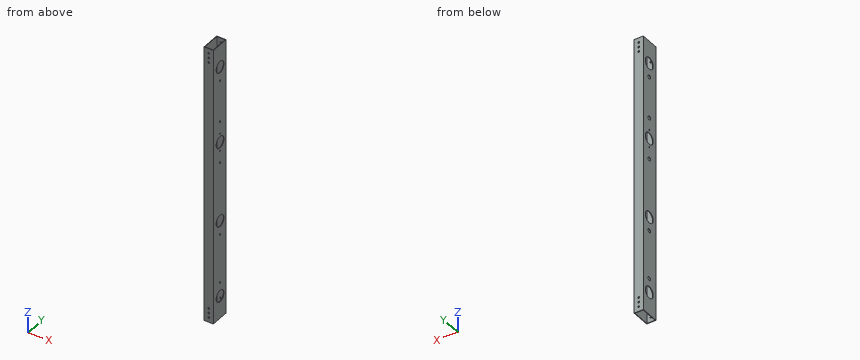
Autodesk Inventor part; units mm, degrees
ref_plane "YZ Plane" through (0, 0, 0) normal (1, 0, 0) x (0, 1, 0)
ref_plane "XZ Plane" through (0, 0, 0) normal (0, 1, 0) x (-1, 0, 0)
ref_plane "XY Plane" through (0, 0, 0) normal (0, 0, 1) x (1, 0, 0)
sketch "Sketch1" plane through (0, 0, 0) normal (1, 0, 0) x (0, 1, 0)
  line L0 (25.4, -381) -> (-25.4, -381)
  line L1 (-25.4, -381) -> (-25.4, 381)
  line L2 (-25.4, 381) -> (25.4, 381)
  line L3 (25.4, 381) -> (25.4, -381)
  line L4 (25.4, -381) -> (-25.4, 381) construction
  line L5 (-25.4, -381) -> (25.4, 381) construction
  circle A0 centre (1.5875, -319.0875) radius 15.875
  line L6 (0, -381) -> (0, -205.8364) construction
  circle A1 centre (1.5875, -280.9875) radius 2.4892
  circle A2 centre (1.5875, -280.9875) radius 5.2705
  circle A3 centre (-1.5875, 0) radius 15.875
  line L7 (0, 0) -> (48.0139, 0) construction
  circle A4 centre (1.5875, 319.0875) radius 15.875
  circle A5 centre (1.5875, 280.9875) radius 2.4892
  circle A6 centre (1.5875, 280.9875) radius 5.2705
  circle A7 centre (1.5875, -319.0875) radius 76.2 construction
  circle A8 centre (-1.5875, 0) radius 76.2 construction
  circle A9 centre (1.5875, 319.0875) radius 76.2 construction
  circle A10 centre (-1.5875, -23.8125) radius 2.0193
  circle A11 centre (19.0347, -11.9063) radius 2.0193
  circle A12 centre (19.0347, 11.9062) radius 2.0193
  circle A13 centre (-1.5875, 23.8125) radius 2.0193
  circle A14 centre (-22.2097, 11.9062) radius 2.0193 construction
  circle A15 centre (-22.2097, -11.9063) radius 2.0193 construction
  circle A16 centre (-1.5875, -57.15) radius 2.4892
  circle A17 centre (-1.5875, -57.15) radius 5.2705
  circle A18 centre (-1.5875, 57.15) radius 2.4892
  circle A19 centre (-1.5875, 57.15) radius 5.2705
  circle A20 centre (1.5875, -109.5375) radius 15.875
  circle A21 centre (1.5875, -147.6375) radius 2.4892
  circle A22 centre (1.5875, -147.6375) radius 5.2705
  line L8 (1.5875, 280.9875) -> (1.5875, 319.0875) construction
  line L9 (1.5875, -109.5375) -> (1.5875, -147.6375) construction
  circle A23 centre (1.5875, 85.725) radius 2.0193
  circle A24 centre (1.5875, 52.3875) radius 2.4892
  circle A25 centre (1.5875, 52.3875) radius 5.2705
  circle A26 centre (1.5875, 166.6875) radius 2.4892
  circle A27 centre (1.5875, 166.6875) radius 5.2705
  circle A28 centre (1.5875, 133.35) radius 2.0193
  line L10 (1.5875, 133.35) -> (1.5875, 85.725) construction
  line L11 (-1.5875, 23.8125) -> (-1.5875, -23.8125) construction
  line L12 (1.5875, 166.6875) -> (1.5875, 52.3875) construction
  line L13 (-1.5875, 57.15) -> (-1.5875, -57.15) construction
  circle A29 centre (1.5875, 109.5375) radius 15.875
  line L14 (25.4, 381) -> (-25.4, 381) construction
  line L15 (-25.4, 381) -> (-25.4, 406.4) construction
  line L16 (-25.4, 406.4) -> (25.4, 406.4) construction
  line L17 (25.4, 406.4) -> (25.4, 381) construction
  line L18 (25.4, 404.8125) -> (-25.4, 404.8125) construction
  line L19 (25.4, 401.6375) -> (-25.4, 401.6375) construction
  point P0 (0, 0)
  point P1 (1.5875, 1.5875)
  point P2 (1.5875, -19.5792)
  point P3 (3.2385, -19.5792)
  point P4 (1.5875, -19.5792)
  dimension "d0" = 762
  dimension "d1" = 50.8
  dimension "d2" = 31.75
  dimension "d4" = 10.541
  dimension "d5" = 4.9784
  dimension "d6" = 1.5875
  dimension "d7" = 1.5875
  dimension "d8" = 38.1
  dimension "d9" = 319.0875
  dimension "d10" = 152.4
  dimension "d13" = 4.0386
  dimension "d16" = 360
  dimension "d18" = 4.9784
  dimension "d19" = 10.541
  dimension "d20" = 114.3
  dimension "d21" = 47.625
  dimension "d22" = 3.1903
  dimension "d26" = 4.0386
  dimension "d28" = 4.9784
  dimension "d29" = 10.541
  dimension "d33" = 360
  dimension "d35" = 219.075
  dimension "d36" = 209.55
  dimension "d58" = 25.4
  dimension "d59" = 1.5875
  dimension "d60" = 3.175
extrude "Extrusion1" add sketch "Sketch1" along normal mid plane 25.4 contours L0 L1 L2 L3 | A2 | A3 | A6 | A10 | A11 | A12 | A13 | A16 | A17 | A18 A25 | A18 A25 A19 A24 | A25 A18 | A18 A25 A19 | A25 A19 A24 | A22 | A27
sketch "Sketch2" plane through (-12.7, -25.4, -381) normal (0, 0, -1) x (-1, 0, 0)
  line L0 (0, 50.8) -> (-25.4, 50.8)
  line L1 (-25.4, 0) -> (-25.4, 50.8)
  line L2 (0, 50.8) -> (0, 0)
  line L3 (-23.8125, 49.2125) -> (-1.5875, 49.2125)
  line L4 (-1.5875, 49.2125) -> (-1.5875, 1.5875)
  line L5 (-1.5875, 1.5875) -> (-23.8125, 1.5875)
  line L6 (-23.8125, 1.5875) -> (-23.8125, 49.2125)
  line L7 (0, 0) -> (-25.4, 0)
  point P0 (-12.7, 25.4)
  dimension "d23" = 1.5875
extrude "Extrusion2" cut sketch "Sketch2" against normal through all contours L3 L4 L5 L6
sketch "Sketch3" plane through (-12.7, 25.4, 381) normal (0, 1, 0) x (1, 0, 0)
  line L0 (0, 762) -> (25.4, 762)
  line L1 (0, 762) -> (25.4, 762)
  line L2 (12.7, 762) -> (12.7, 749.3)
  circle A0 centre (12.7, 749.3) radius 2.4892
  circle A1 centre (12.7, 736.6) radius 2.4892
  circle A2 centre (12.7, 723.9) radius 2.4892
  line L3 (12.7, 381) -> (42.3415, 381) construction
  circle A3 centre (12.7, 12.7) radius 2.4892
  circle A4 centre (12.7, 25.4) radius 2.4892
  circle A5 centre (12.7, 38.1) radius 2.4892
  dimension "d37" = 12.7
  dimension "d38" = 4.9784
  dimension "d41" = 12.7
extrude "Extrusion3" cut sketch "Sketch3" against normal through all
sketch "Sketch4" plane through (-12.7, 0, 0) normal (-1, 0, 0) x (0, 0, 1)
  circle A0 centre (280.9875, 1.5875) radius 2.4892
  circle A1 centre (-280.9875, 1.5875) radius 2.4892
  circle A2 centre (52.3875, 1.5875) radius 2.4892
  circle A3 centre (166.6875, 1.5875) radius 2.4892
  circle A4 centre (-147.6375, 1.5875) radius 2.4892
  point P0 (0, 0)
  point P1 (57.15, -1.5875)
hole "Hole1" at (-12.7, 1.5875, 280.9875) at (-12.7, 1.5875, 52.3875) at (-12.7, 1.5875, 166.6875) at (-12.7, 1.5875, -280.9875) at (-12.7, 1.5875, -147.6375) direction (1, 0, 0) diameter 4.9784 depth 25.4 tip angle 118 counterbore diameter 10.541 counterbore depth 4.826
equation "\"d7\" = d6"
properties part number "VersaChassis Drive Rail Template" material "Aluminum"
CAD build for the part. Positions are in the model's coordinates, mm. Round coordinates to 2 decimals unless told otherwise and drop trailing zeros. Order: outer loops, then holes, each group sorted by start corner. A loop starts at its lowest first (then second) coordinate and runs counter-clockwise, first axis right, second up. Notation, with made-up numbers: (12, 6.5) - (46, 6.5) arc R15 ccw to (46, 16.5) - close; hole circle Ø7 at (-10.5, -19.5). An arc over 180 degrees is marked (long way). Answer in a Markdown table with one row per item. Add a question column.
(1) Drop flat-ended pins along their axis: pin 1 Ø4 at (y, z) = (0.5, -145.5) entering from +X; pin 2 Ø5.5 at (y, z) = (1.59, 166.69) entering from -X. Give the stop position or say it passes through.
(2) Probe L1, parallel to Y at x = -11, z = 141; L2, parallel to X at y = -7.5, z = 64.5; L3, parallel to X at y = -24.15, z = 355.6. List the from-to ranges inside material, lowest first. Write a range as [from, to].
(3) Band-saw the part on A-A on z = 8.5. List the corners of the cut face in (x, y), and give its area (3 significant figures).
Data:
| question | item | result |
|---|---|---|
| 1 | pin 1 | stops at x = 12.7 |
| 1 | pin 2 | stops at x = 11.11 |
| 2 | L1 | y = [-25.4, -23.81], [23.81, 25.4] |
| 2 | L2 | x = [-12.7, -11.11], [11.11, 12.7] |
| 2 | L3 | x = [-12.7, -2.49], [2.49, 12.7] |
| 3 | outline | (-12.7, -25.4) - (12.7, -25.4) - (12.7, 25.4) - (-12.7, 25.4) - close; hole (-11.11, -23.81) - (11.11, -23.81) - (11.11, 23.81) - (-11.11, 23.81) - close |
| 3 | area | 232 mm^2 |
